Here's how the part is built. I have some questions about the finished solid (model axes, mm). Round coordinates to 2 decimals unless told otherwise and drop trailing zeros. Order: outer loops, then holes, each group sorted by start corner. A loop starts at its lowest first (then second) coordinate and runs counter-clockwise, first axis right, second up. Notation, with made-up numbers: (-10, -16) -> (23, -16) arc R27 cw to (23, 10) -> close; hole circle Ø7 at (-22.5, -12.5). An arc over 180 degrees is marked (long way). Use a Markdown table: item, result. Add a question column.
from build123d import *

# Parameters (mm, degrees)
F0_W     = 50
F0_H     = 50
F1_DEPTH = 1000
F3_DEPTH = 50
F4_R     = 17.5
F5_DEPTH = 3
F6_R     = 17.5
F7_DEPTH = 3


with BuildPart() as f1:
    # F0 (on Top) → F1 (new body)
    with BuildSketch(Plane.XY):
        with Locations((0, 2.417763)):
            Rectangle(F0_W, F0_H)
    extrude(amount=F1_DEPTH)

    # F2 (on face) → F3 (join)
    with BuildSketch(Plane.XZ.offset(22.582237)):
        Polygon((-25, 1000), (25, 1000), (325, 1000), (325, 1200), (-325, 1200), (-325, 1000), align=None)
        Polygon((25, 1040), (-295, 1040), (-295, 1160), (295, 1160), (295, 1040), align=None, mode=Mode.SUBTRACT)
    extrude(amount=-F3_DEPTH)

    # F4 (on face) → F5 (join)
    with BuildSketch(Plane.YZ.offset(25)):
        with Locations((0, 50)):
            Circle(F4_R)
    extrude(amount=F5_DEPTH)

    # F6 (on face) → F7 (join)
    with BuildSketch(Plane(origin=(-25, 0, 0), x_dir=(0, -1, 0), z_dir=(-1, 0, 0))):
        with Locations((-2.417763, 50)):
            Circle(F6_R)
    extrude(amount=F7_DEPTH)


solid = f1.part
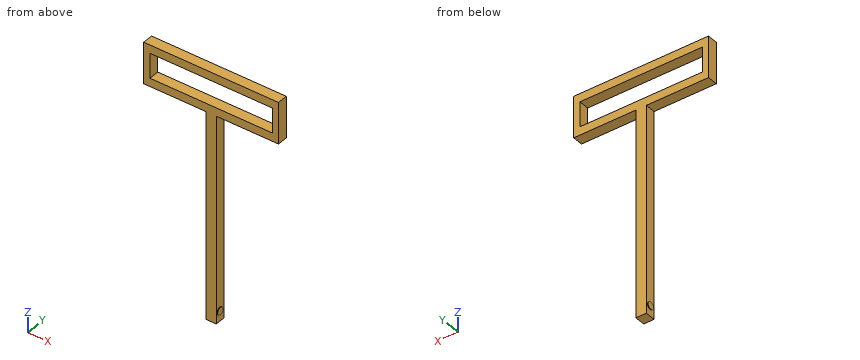
(1) Please list where these lines run through material, in increasing order: probe 1 along Z at (x, y) = (192, -3); probe 2 along Z at (x, y) = (-7.5, -14); probe 3 along X at (y, z) = (7, 964). Write a range as from..to.
(2) I want a section at A-A on x = 2. List the corners of the cut face in (y, z) for me.
(3) I want a section at B-B on y = 0. List the corners of the cut face in (x, z) for me, and give its area (3 significant figures).
(4) I want a section at C-C on z = 50. List the corners of the cut face in (x, y) for me.
(5) I'm going to push flat-ended pins straight in: P1, Ø4, axis at y = 15.5, z = 580, coming from the +X side; P2, Ø25, axis at x = -166.5, y = -2.5, coming from the -Z side; P3, Ø6, axis at y = 21, z = 278, coming from the -X side. Where does each tip first touch, or does it pass through?
Output:
| question | item | result |
|---|---|---|
| 1 | probe 1 | 1000..1040, 1160..1200 |
| 1 | probe 2 | 0..1040, 1160..1200 |
| 1 | probe 3 | -25..25 |
| 2 | outline | (-22.58, 0) -> (27.42, 0) -> (27.42, 1040) -> (-22.58, 1040) -> close; (-22.58, 1160) -> (27.42, 1160) -> (27.42, 1200) -> (-22.58, 1200) -> close |
| 3 | outline | (-325, 1000) -> (-25, 1000) -> (-25, 67.33) -> (-28, 67.33) -> (-28, 32.67) -> (-25, 32.67) -> (-25, 0) -> (25, 0) -> (25, 32.5) -> (28, 32.5) -> (28, 67.5) -> (25, 67.5) -> (25, 1000) -> (325, 1000) -> (325, 1200) -> (-325, 1200) -> close; hole (-295, 1040) -> (295, 1040) -> (295, 1160) -> (-295, 1160) -> close |
| 3 | area | 109,000 mm² |
| 4 | outline | (-28, -15.08) -> (-25, -15.08) -> (-25, -22.58) -> (25, -22.58) -> (25, -17.5) -> (28, -17.5) -> (28, 17.5) -> (25, 17.5) -> (25, 27.42) -> (-25, 27.42) -> (-25, 19.92) -> (-28, 19.92) -> close |
| 5 | P1 | x = 25 |
| 5 | P2 | z = 1000 |
| 5 | P3 | x = -25 |
